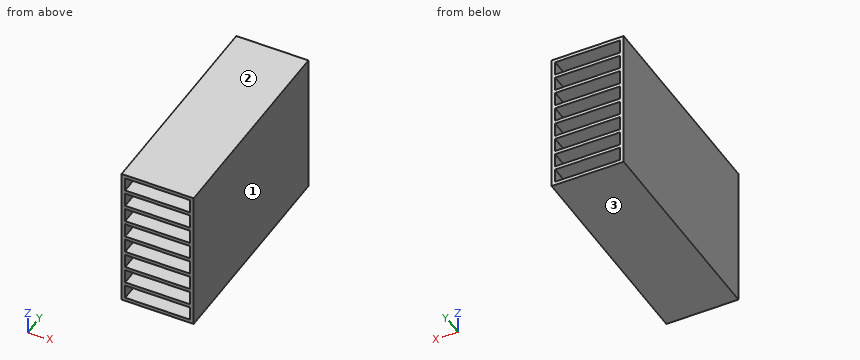
```python
from build123d import *

# Parameters (mm, degrees)
ESQUISSE1_W             = 60
ESQUISSE1_H             = 40
BOSS_EXTRU_1_DEPTH      = 20
ESQUISSE2_W             = 18
ESQUISSE2_H             = 3.875
ENL_V_MAT_EXTRU_1_DEPTH = 67.332495807


with BuildPart() as part:
    # Esquisse1 → Boss.-Extru.1 (new body)
    with BuildSketch(Plane.YZ):
        Rectangle(ESQUISSE1_W, ESQUISSE1_H)
    extrude(amount=BOSS_EXTRU_1_DEPTH)

    # Esquisse2 → Enlèv. mat.-Extru.1 (cut, through all)
    with BuildSketch(Plane.XZ.offset(30)):
        with Locations((10, 17.0625)):
            Rectangle(ESQUISSE2_W, ESQUISSE2_H)
        with Locations((10, 12.1875)):
            Rectangle(ESQUISSE2_W, ESQUISSE2_H)
        with Locations((10, 7.3125)):
            Rectangle(ESQUISSE2_W, ESQUISSE2_H)
        with Locations((10, 2.4375)):
            Rectangle(ESQUISSE2_W, ESQUISSE2_H)
        with Locations((10, -2.4375)):
            Rectangle(ESQUISSE2_W, ESQUISSE2_H)
        with Locations((10, -7.3125)):
            Rectangle(ESQUISSE2_W, ESQUISSE2_H)
        with Locations((10, -12.1875)):
            Rectangle(ESQUISSE2_W, ESQUISSE2_H)
        with Locations((10, -17.0625)):
            Rectangle(ESQUISSE2_W, ESQUISSE2_H)
    extrude(amount=-ENL_V_MAT_EXTRU_1_DEPTH, mode=Mode.SUBTRACT)


solid = part.part
```
Could you check a few things on this model? Use its own coordinates, in mm. Face numbers are marked on the shaded views. Round coordinates to 2 decimals unless told otherwise and drop trailing zeros. Loops run counter-clockwise (first coordinate to the right, second up) from the corner with the lowest first, then second, coordinate; pieces in that order, holes last. Notation, with made-up numbers: (55.5, 34.5) - (112.5, 34.5) arc R34 cw to (112.5, 71.5) - close; hole circle Ø5 at (48.5, -38.5). An arc over 180 degrees is marked (long way). Answer in a Markdown table with one row per item. Add a question column.
(1) If we section it at A-A (z = -8.5): Please give me the cut outline in (x, y), plus the area to 3 significant figures.
(2) If we mould it in two halves opening along Z, with no side actions, what happens to the marked faces 1, 2 and 3? For each: pulls with the +Z half, pulls with the -Z half, needs draft (parallel to the pull), parting line crosses it, or undercut.
(3) If we section it at B-B (x = 4.75): State how many separate pieces and enclosed holes the cut face has, plus the area to 3 significant figures.
(4) I need wall thicknesses on line 1 along X through (y, z) = (7.5, -17). Which ranges of the line are inside material? Lowest first, please.
Model answer:
| question | item | result |
|---|---|---|
| 1 | outline | (0, -30) - (1, -30) - (1, 30) - (0, 30) - close; (19, -30) - (20, -30) - (20, 30) - (19, 30) - close |
| 1 | area | 120 mm² |
| 2 | face 1 | needs draft |
| 2 | face 2 | pulls with the +Z half |
| 2 | face 3 | pulls with the -Z half |
| 3 | separate pieces | 9 |
| 3 | enclosed holes | 0 |
| 3 | area | 540 mm² |
| 4 | line 1 | x = 0 to 1, 19 to 20 |
